Part model, mm, in its own coordinate system. Face numbers are marked on the shaded views. A direction names the side the tool comes from. Coordinates: 2 decimals unless noted, no trailing zeros. Loops run counter-clockwise (first coordinate to the right, second up) from the corner with the lowest first, then second, coordinate; pieces in that order, holes last. Notation, with made-up numbers: (11, 75.25) - (61, 75.25) arc R19 ccw to (61, 102.25) - close; hole circle Ø11 at (39, 79). An arc over 180 degrees is marked (long way). One line per question, with ' | ' between items. Start each with the question number.
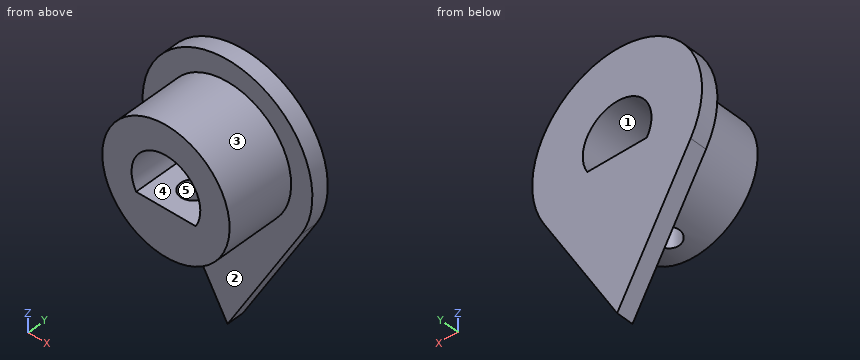
from build123d import *

# Parameters (mm, degrees)
SKETCH_1_R          = 7.5
SKETCH_1_R_2        = 4.05
EXTRUDE_1_DEPTH     = 10
EXTRUDE_START       = -2
SKETCH_2_R          = 4.05
EXTRUDE_2_DEPTH     = 2
EXTRUDE_3_DEPTH     = 10
SKETCH_4_R          = 1.45
CUT_EXTRUDE_1_DEPTH = 10


with BuildPart() as part:
    # 草图1 → 凸台-拉伸1 (new body)
    with BuildSketch(Plane(origin=(0, 0, 0), x_dir=(1, 0, 0), z_dir=(0, 1, 0))):
        with Locations(Location((0, 0, 0), (0, 0, 270))):
            Circle(SKETCH_1_R)
        with Locations(Location((0, 0, 0), (0, 0, 270))):
            Circle(SKETCH_1_R_2, mode=Mode.SUBTRACT)
    extrude(amount=EXTRUDE_1_DEPTH)

    # 草图2 → 凸台-拉伸2 (add)
    with BuildSketch(Plane(origin=(0, 10, 0), x_dir=(1, 0, 0), z_dir=(0, 1, 0)).offset(EXTRUDE_START)):
        with BuildLine():
            Line((-8.660254038, 5), (0, 20))
            Line((0, 20), (8.660254038, 5))
            ThreePointArc((8.660254038, 5), (0, -10), (-8.660254038, 5))
        make_face()
        with Locations(Location((0, 0, 0), (0, 0, 270))):
            Circle(SKETCH_2_R, mode=Mode.SUBTRACT)
    extrude(amount=EXTRUDE_2_DEPTH)

    # 草图3 → 凸台-拉伸3 (add)
    with BuildSketch(Plane.XZ):
        with BuildLine():
            Line((-3.507402885, -2.025), (3.507402885, -2.025))
            ThreePointArc((3.507402885, -2.025), (0, -4.05), (-3.507402885, -2.025))
        make_face()
    extrude(amount=-EXTRUDE_3_DEPTH)

    # 草图4 → 切除-拉伸1 (cut)
    with BuildSketch(Plane.XY):
        with Locations((0, 3.5)):
            Circle(SKETCH_4_R)
    extrude(amount=-CUT_EXTRUDE_1_DEPTH, mode=Mode.SUBTRACT)


solid = part.part
1) Wall check: line 1 along X through (y, z) = (6.5, 0); line 2 along Y through (x, z) = (0, -3.25); line 3 along Z through (x, y) = (0, 5.5) (3 decimals). Give the ranges that are in metal, low to high. Write a range as [from, to].
2) Tool access for the marked faces 1 and 2: list every direction of +Z, -Z, +X, -X, +Y, -Y with a clear straight run to the whole face (end or side of a thin tool).
3) Mould opens along Z. For the marked faces 3, 4 and 5 say: +Z half, -Z half, draft (parallel to the pull), parting line (faces both ways), or undercut.
4) Band-saw the part on B-B on x = 4.75. List the corners of the cut face in (y, z).
5) Band-saw the part on A-A on z = 0. List the corners of the cut face in (x, y).
6) Band-saw the part on C-C on y = 1. List the corners of the cut face in (x, z) (3 decimals), then the cut area to 3 significant figures.
7) Band-saw the part on D-D on z = 7. List the corners of the cut face in (x, y).
8) Pin check, flat tips, straight feed: pin 1 Ø1.5 at (y, z) = (8.5, -11) entering from +X; pin 2 Ø5.5 at (x, y) = (0, 4.5) entering from +Z; pin 3 Ø1 at (x, y) = (-7, 3) entering from +Z. Stop position of each tip, or through.
Values found:
1) line 1: [-7.5, -4.05], [4.05, 7.5] | line 2: [0, 2.05], [4.95, 10] | line 3: [-7.5, -2.025], [4.05, 7.5]
2) face 1: +Y, -Y | face 2: -Y
3) face 3: parting line | face 4: undercut | face 5: draft
4) outline: (0, -5.8) - (8, -5.8) - (8, -11.77) - (10, -11.77) - (10, 8.8) - (8, 8.8) - (8, 5.8) - (0, 5.8) - close
5) outline: (-10, 8) - (-7.5, 8) - (-7.5, 0) - (-4.05, 0) - (-4.05, 10) - (-10, 10) - close; (4.05, 0) - (7.5, 0) - (7.5, 8) - (10, 8) - (10, 10) - (4.05, 10) - close
6) outline: circle Ø15 at (0, 0); hole (-3.507, -2.025) - (3.507, -2.025) arc R4.05 ccw (long way) to start | area: 135 mm²
7) outline: (-7.14, 8) - (-2.69, 8) - (-2.69, 0) - (2.69, 0) - (2.69, 8) - (7.14, 8) - (7.14, 10) - (-7.14, 10) - close
8) pin 1: x = 5.63 | pin 2: z = 7.5 | pin 3: z = 3.74
